Here's how the part is built. I have some questions about the finished solid (model axes, mm). A direction names the side the tool comes from. Round coordinates to 2 decimals unless told otherwise and drop trailing zeros. Write each loop counter-clockwise with the first axis right and the second up, starting at its lowest first coordinate (ties: lowest second). Pieces come first, ordered by that corner, then holes. Notation, with made-up numbers: (5, -12) - (40, -12) arc R32 cw to (40, 19) - close; hole circle Ø7 at (-3, 66). An arc over 180 degrees is marked (long way). Use one line per item in the form item = value. Start each with the question number.
1. We'd pull the mould along X, two halves only. Please class faces 1 (the flat face through (-8.1, 2, 0)), 2 (the flat face through (3.09, 1.97, -5.26)), 3 (the flat face through (0, 2, 11.044)): +X half, -X half, draft (parallel to the pull), parting line (faces both ways), or undercut.
2. I want a section at A-A, the plane z = -0.5. List the corners of the cut face in (x, y) for me.
3. I want a section at B-B, the plane y = 1. List the corners of the cut face in (x, z) for me, plus the area to 3 significant figures.
4. I want a section at C-C, the plane x = -4.5. List the corners of the cut face in (y, z) for me, plus the area to 3 significant figures.
5. If I drill on line 1 along X through (y, z) = (3.5, -1); line 2 along Z through (x, y) = (-3.25, 0.95); line 3 along Z through (x, y) = (3, 2.2), over which ranges is the centre line in solid material (lowest first)?
6. Which directions (+Z, -Z, +X, -X, +Y, -Y) give clear straight access to the entire face, cutting with the end or side of a thin tool? Please do faces 4 (the flat face through (-3.007, 1.972, -5.307)), 5 (the flat face through (0, 2, -11.044)).
```python
from build123d import *

# Parameters (mm, degrees)
EXTRUDE_1_DEPTH = 4


with BuildPart() as part:
    # 草图1 → 凸台-拉伸1 (new body)
    with BuildSketch(Plane(origin=(0, 0, 0), x_dir=(1, 0, 0), z_dir=(0, 1, 0))):
        Polygon((-8.1, 4.67653718), (-8.1, -4.67653718), (-8.1, -11.043673284), (8.1, -11.043673284), (8.1, -4.67653718), (8.1, 4.67653718), (8.1, 11.043673284), (-8.1, 11.043673284), align=None)
        Polygon((0, 7.043673284), (-6.1, 3.521836642), (-6.1, -3.521836642), (0, -7.043673284), (6.1, -3.521836642), (6.1, 3.521836642), align=None, mode=Mode.SUBTRACT)
    extrude(amount=EXTRUDE_1_DEPTH)


solid = part.part
```
Model answer:
q1.face_1 = -X half
q1.face_2 = undercut
q1.face_3 = draft
q2.outline = (-8.1, 0) - (-6.1, 0) - (-6.1, 4) - (-8.1, 4) - close; (6.1, 0) - (8.1, 0) - (8.1, 4) - (6.1, 4) - close
q3.outline = (-8.1, -11.04) - (8.1, -11.04) - (8.1, 11.04) - (-8.1, 11.04) - close; hole (-6.1, -3.52) - (0, -7.04) - (6.1, -3.52) - (6.1, 3.52) - (0, 7.04) - (-6.1, 3.52) - close
q3.area = 229 mm2
q4.outline = (0, -11.04) - (4, -11.04) - (4, -4.45) - (0, -4.45) - close; (0, 4.45) - (4, 4.45) - (4, 11.04) - (0, 11.04) - close
q4.area = 52.8 mm2
q5.line_1 = -8.1 to -6.1, 6.1 to 8.1
q5.line_2 = -11.04 to -5.17, 5.17 to 11.04
q5.line_3 = -11.04 to -5.31, 5.31 to 11.04
q6.face_4 = +Y, -Y
q6.face_5 = -Z, +X, -X, +Y, -Y
